```python
from build123d import *

# Parameters (mm, degrees)
F0_R     = 90.5
F1_DEPTH = 41.1


with BuildPart() as f1:
    # F0 (on Top) → F1 (new body)
    with BuildSketch(Plane.XY):
        with Locations((-117.5, 0)):
            Circle(F0_R)
    extrude(amount=F1_DEPTH)

    # F2 (on Front) → F3 (revolve, cut)
    with BuildSketch(Plane.XZ):
        with BuildLine():
            Line((-189.314945, 33.667415), (-186.16, 41.1))
            Line((-186.16, 41.1), (-198.07, 41.1))
            Line((-198.07, 41.1), (-194.915055, 33.667415))
            ThreePointArc((-194.915055, 33.667415), (-194.620201, 33.312891), (-194.178651, 33.18))
            Line((-194.178651, 33.18), (-190.051349, 33.18))
            ThreePointArc((-190.051349, 33.18), (-189.609799, 33.312891), (-189.314945, 33.667415))
        make_face()
        with BuildLine():
            ThreePointArc((-189.314945, 7.432585), (-189.609799, 7.787109), (-190.051349, 7.92))
            Line((-190.051349, 7.92), (-194.178651, 7.92))
            ThreePointArc((-194.178651, 7.92), (-194.620201, 7.787109), (-194.915055, 7.432585))
            Line((-194.915055, 7.432585), (-198.07, 0))
            Line((-198.07, 0), (-186.16, 0))
            Line((-186.16, 0), (-189.314945, 7.432585))
        make_face()
    revolve(axis=Axis((-117.5, 0, 20.55), (0, 0, -1)), mode=Mode.SUBTRACT)


solid = f1.part
```
Can you work these out from the model? Positions are in its coordinate system, mm. A direction names the side the tool comes from. Round coordinates to 2 decimals unless told otherwise and drop trailing zeros. Order: outer loops, then holes, each group sorted by start corner. A loop starts at its lowest first (then second) coordinate and runs counter-clockwise, first axis right, second up.
(1) On a 3-axis mill with a long thin cutter (end or side, diameter ignored), from which of +Z, -Z, +X, -X, +Y, -Y can I reach the whole of each face in a straight line? I mean faces 1 (the face through (-174, 46, 33.18)), 2 (the face through (-61, 46, 7.92)), 3 (the face through (-178.3, -53.2, 0)). Say none if no direction works.
Results are:
face 1: +Z
face 2: -Z
face 3: -Z, +X, -X, +Y, -Y
(2) If we section it at A-A (x = -117.5): Please give me the cut outline in (y, z), plus the area to 3 significant figures.
Results are:
outline: (-90.5, 0) - (-80.57, 0) - (-77.42, 7.43) arc R0.8 cw to (-76.68, 7.92) - (-72.55, 7.92) arc R0.8 cw to (-71.81, 7.43) - (-68.66, 0) - (68.66, 0) - (71.81, 7.43) arc R0.8 cw to (72.55, 7.92) - (76.68, 7.92) arc R0.8 cw to (77.42, 7.43) - (80.57, 0) - (90.5, 0) - (90.5, 41.1) - (80.57, 41.1) - (77.42, 33.67) arc R0.8 cw to (76.68, 33.18) - (72.55, 33.18) arc R0.8 cw to (71.81, 33.67) - (68.66, 41.1) - (-68.66, 41.1) - (-71.81, 33.67) arc R0.8 cw to (-72.55, 33.18) - (-76.68, 33.18) arc R0.8 cw to (-77.42, 33.67) - (-80.57, 41.1) - (-90.5, 41.1) - close
area: 7,170 mm2
(3) If we section it at B-B (y = 0): Please give me the cut outline in (x, z), plus the area to 3 significant figures.
Results are:
outline: (-208, 0) - (-198.07, 0) - (-194.92, 7.43) arc R0.8 cw to (-194.18, 7.92) - (-190.05, 7.92) arc R0.8 cw to (-189.31, 7.43) - (-186.16, 0) - (-48.84, 0) - (-45.69, 7.43) arc R0.8 cw to (-44.95, 7.92) - (-40.82, 7.92) arc R0.8 cw to (-40.08, 7.43) - (-36.93, 0) - (-27, 0) - (-27, 41.1) - (-36.93, 41.1) - (-40.08, 33.67) arc R0.8 cw to (-40.82, 33.18) - (-44.95, 33.18) arc R0.8 cw to (-45.69, 33.67) - (-48.84, 41.1) - (-186.16, 41.1) - (-189.31, 33.67) arc R0.8 cw to (-190.05, 33.18) - (-194.18, 33.18) arc R0.8 cw to (-194.92, 33.67) - (-198.07, 41.1) - (-208, 41.1) - close
area: 7,170 mm2
(4) I'm going to push flat-ended pins straight in: pin 1 (2 mm diameter, centred on x = -189, z = 28.5, fed in from -Y); pin 2 (1.5 mm diameter, centred on y = -72, z = 26, fed in from +X); pin 3 (6 mm diameter, centred on y = -64, z = 27.5, fed in from -X). Where does each tip first touch, or does it pass through?
Results are:
pin 1: stops at y = -56.75
pin 2: stops at x = -61.7
pin 3: stops at x = -184.35
(5) If we section it at C-C (z = 24.5): Please give me the cut outline in (x, y), plus the area to 3 significant figures.
Results are:
outline: circle Ø181 at (-117.5, 0)
area: 25,700 mm2
(6) If I drill on L1, parallel to Y at x = -57.5, z = 35.5; L2, parallel to X at y = -44, z = 34; L3, parallel to X at y = -56, z = 2, over which ranges is the centre line in solid material (lowest first)?
Results are:
L1: y = -67.75 to -50.14, -38.03 to 38.03, 50.14 to 67.75
L2: x = -196.58 to -181.37, -174.08 to -60.92, -53.63 to -38.42
L3: x = -188.59 to -174.24, -158.68 to -76.32, -60.76 to -46.41
(7) We'd pull the mould along X, two halves only. Please class faces 4 (the face through (-62.86, -41.9, 0.46)), 5 (the face through (-31.18, 27.18, 20.26)), 6 (the face through (-178.3, -53.2, 41.1)), 7 (the face through (-181.066, -26.356, 40.739)): +X half, -X half, draft (parallel to the pull), parting line (faces both ways), or undercut.
Results are:
face 4: undercut
face 5: parting line
face 6: draft
face 7: undercut
